Verification items for the finished model (mm, model axes). A direction names the side the tool comes from. Round coordinates to 2 decimals unless told otherwise and drop trailing zeros. Write each loop counter-clockwise with the first axis right and the second up, starting at its lowest first coordinate (ties: lowest second). Pieces come first, ordered by that corner, then holes. Notation, with made-up numbers: M 70,23 L 110,23 A8 cw 110,36 Z; hole C 54,68.25 d8. An arc over 180 degrees is marked long. One line per item, written item: value. Start each with the question number.
Item 1: Section check D-D, the plane z = -13.5. Record the cut outline in (x, y), then the cut area to 3 significant figures.
Item 2: Section check A-A, the plane y = 5.5. Record the cut outline in (x, z).
Item 3: Draft check along Z on faces 5 (the face through (10.99, 28.29, 20.64)), 6 (the face through (14, -14, 21)), 7 (the face through (5, -31, -17.35)). Enter one of: +Z half, -Z half, draft (parallel to the pull), parting line (faces both ways), or undercut.
Item 4: Gauge pin test, flat ends, axial feed: pin 1 (1 mm diameter, centred on y = 4, z = -8.5, fed in from +X); pin 2 (5 mm diameter, centred on x = 9.5, z = -18.5, fed in from -Y); pin 3 (1.4 mm diameter, centred on x = 7, z = 21.5, fed in from +Y); pin 4 (6 mm diameter, centred on y = -30.5, z = -21, fed in from -X). Record the tip position at first contact, or that the pin passes through.
Item 5: Tool access check on faces 1 (the face through (10.4, -30.4, 10.9)), 2 (the face through (10, 29.2, 21.4)), 3 (the face through (7, 31, -7)), 4 (the face through (7, 10, -3.9)). Record the directions out of +Z, -Z, +X, -X, +Y, -Y that give a thin tool (end or side, any length) a straight path to the whole face; none if there is none.
Item 6: Section check C-C, the plane y = 13.59. Record the cut outline in (x, z).
Item 7: Section check B-B, the plane z = 10.9. Record the cut outline in (x, y).
Item 8: Thickness scan on probe 1 along Y at (x, z) = (7.75, -8.5); probe 2 along Z at (x, y) = (4.5, 2); probe 3 along Z at (x, y) = (3.75, 12). Record the ranges inside material, lowest first. Write a range as from..to.
from build123d import *

# Parameters (mm, degrees)
SKETCH_1_W           = 46
SKETCH_1_H           = 64
EXTRUDE_1_DEPTH      = 12
SHELL_1_T            = -2
SKETCH_3_W           = 4.4
SKETCH_3_H           = 2
SKETCH_3_W_2         = 3.9
SKETCH_3_H_2         = 18.35
EXTRUDE_6_DEPTH      = 10
SKETCH_4_R           = 1
CUT_EXTRUDE_1_DEPTH  = 10
CUT_EXTRUDE_3_REACH  = 43.195
SKETCH_7_R           = 1
EXTRUDE_START        = -12
SKETCH_8_R           = 0.9
EXTRUDE_7_DEPTH      = 2
SKETCH_13_W          = 24
SKETCH_13_H          = 1.25
EXTRUDE_8_DEPTH      = 12
CUT_EXTRUDE_4_REACH  = 71.433
CUT_EXTRUDE_5_REACH  = 71.433
CUT_EXTRUDE_START    = -4
CUT_EXTRUDE_6_DEPTH  = 2.1
CUT_EXTRUDE_START_2  = -1.5
CUT_EXTRUDE_7_DEPTH  = 30.1
CUT_EXTRUDE_8_REACH  = 59.758
CUT_EXTRUDE_9_REACH  = 71.433
SKETCH_15_W          = 10
SKETCH_15_H          = 6
CUT_EXTRUDE_10_REACH = 59.758
SKETCH_16_W          = 1.6
SKETCH_16_H          = 6.7


with BuildPart() as part:
    # 草图1 → 凸台-拉伸1 (new body)
    with BuildSketch(Plane(origin=(0, 0, 0), x_dir=(0, 0, -1), z_dir=(1, 0, 0))):
        Rectangle(SKETCH_1_W, SKETCH_1_H)
    extrude(amount=EXTRUDE_1_DEPTH)

    # 抽壳1
    shell_1_openings = [part.faces().sort_by_distance(p)[0] for p in [
        (12, 0, 0),
    ]]
    offset(amount=SHELL_1_T, openings=shell_1_openings, kind=Kind.INTERSECTION)

    # 草图3 → 凸台-拉伸6 (add)
    # profile 1 of 5: a face of its own
    with BuildSketch(Plane(origin=(2, 0, 0), x_dir=(0, 0, -1), z_dir=(1, 0, 0))):
        with BuildLine():
            Line((20.175, -24.35), (21, -24.35))
            Line((21, -24.35), (21, -30))
            Line((21, -30), (15.35, -30))
            Line((15.35, -30), (15.35, -29.175))
            ThreePointArc((15.35, -29.175), (16.763209781, -25.763209781), (20.175, -24.35))
        make_face()
    # profile 2 of 5: a face of its own
    with BuildSketch(Plane(origin=(2, 0, 0), x_dir=(0, 0, -1), z_dir=(1, 0, 0))):
        with Locations((18.8, 1.6)):
            Rectangle(SKETCH_3_W, SKETCH_3_H)
    # profile 3 of 5: a face of its own
    with BuildSketch(Plane(origin=(2, 0, 0), x_dir=(0, 0, -1), z_dir=(1, 0, 0))):
        with BuildLine():
            Line((-21, 30), (-21, 24.35))
            Line((-21, 24.35), (-20.175, 24.35))
            ThreePointArc((-20.175, 24.35), (-17.207572663, 25.370397524), (-15.495256417, 28))
            Line((-15.495256417, 28), (-2, 28))
            Line((-2, 28), (-2, -2.35))
            Line((-2, -2.35), (5.9, -2.35))
            Line((5.9, -2.35), (5.9, 0.6))
            Line((5.9, 0.6), (10.4, 0.6))
            Line((10.4, 0.6), (10.4, 2.6))
            Line((10.4, 2.6), (5.9, 2.6))
            Line((5.9, 2.6), (5.9, 21.5))
            Line((5.9, 21.5), (0, 21.5))
            Line((0, 21.5), (0, 30))
            Line((0, 30), (-21, 30))
        make_face()
        with Locations((1.95, 10.325)):
            Rectangle(SKETCH_3_W_2, SKETCH_3_H_2, mode=Mode.SUBTRACT)
    # profile 4 of 5: a face of its own
    with BuildSketch(Plane(origin=(2, 0, 0), x_dir=(0, 0, -1), z_dir=(1, 0, 0))):
        with BuildLine():
            Line((-21, -10.7), (-21, -16.7))
            ThreePointArc((-21, -16.7), (-18, -13.7), (-21, -10.7))
        make_face()
    # profile 5 of 5: a face of its own
    with BuildSketch(Plane(origin=(2, 0, 0), x_dir=(0, 0, -1), z_dir=(1, 0, 0))):
        with BuildLine():
            Line((18.75, 30), (21, 30))
            Line((21, 30), (21, 27.9))
            Line((21, 27.9), (20.192225279, 27.9))
            ThreePointArc((20.192225279, 27.9), (19.145277228, 28.72622473), (18.75, 30))
        make_face()
    extrude(amount=EXTRUDE_6_DEPTH)

    # 草图4 → 切除-拉伸1 (cut)
    # profile 1 of 2: a face of its own
    with BuildSketch(Plane.ZY):
        with BuildLine():
            Line((-20.175, -26.35), (-23, -26.35))
            Line((-23, -26.35), (-23, -32))
            Line((-23, -32), (-17.382192318, -32))
            Line((-17.382192318, -32), (-17.35, -32))
            Line((-17.35, -32), (-17.35, -29.175))
            ThreePointArc((-17.35, -29.175), (-18.177423343, -27.177423343), (-20.175, -26.35))
        make_face()
        with Locations((-20.175, -29.175)):
            Circle(SKETCH_4_R, mode=Mode.SUBTRACT)
    # profile 2 of 2: a face of its own
    with BuildSketch(Plane.ZY):
        with BuildLine():
            Line((20.175, 26.35), (23, 26.35))
            Line((23, 26.35), (23, 32))
            Line((23, 32), (17.35, 32))
            Line((17.35, 32), (17.35, 29.175))
            ThreePointArc((17.35, 29.175), (18.177423343, 27.177423343), (20.175, 26.35))
        make_face()
        with Locations((20.175, 29.175)):
            Circle(SKETCH_4_R, mode=Mode.SUBTRACT)
    extrude(amount=-CUT_EXTRUDE_1_DEPTH, mode=Mode.SUBTRACT)

    # 草图7 → 切除-拉伸3 (cut, up to next)
    with BuildSketch(Plane.ZY, mode=Mode.PRIVATE) as cut_extrude_3_sk1:
        with Locations((-20.175, -29.175)):
            Circle(SKETCH_7_R)
    cut_extrude_3_tool1 = extrude(cut_extrude_3_sk1.sketch, amount=-CUT_EXTRUDE_3_REACH, mode=Mode.PRIVATE) & part.part
    # 草图7 → 切除-拉伸3 (cut, up to next)
    with BuildSketch(Plane.ZY, mode=Mode.PRIVATE) as cut_extrude_3_sk2:
        with Locations((20.175, 29.175)):
            Circle(SKETCH_7_R)
    cut_extrude_3_tool2 = extrude(cut_extrude_3_sk2.sketch, amount=-CUT_EXTRUDE_3_REACH, mode=Mode.PRIVATE) & part.part
    add(cut_extrude_3_tool1.solids().sort_by_distance((0, -29.175, -20.175))[0], mode=Mode.SUBTRACT)
    add(cut_extrude_3_tool2.solids().sort_by_distance((0, 29.175, 20.175))[0], mode=Mode.SUBTRACT)

    # 草图8 → 凸台-拉伸7 (add)
    with BuildSketch(Plane.ZY.offset(EXTRUDE_START)):
        with Locations(Location((-21, 30, 0), (0, 0, 180))):
            Circle(SKETCH_8_R)
        with Locations(Location((21, -13.7, 0), (0, 0, 180))):
            Circle(SKETCH_8_R)
    extrude(amount=-EXTRUDE_7_DEPTH)

    # 草图13 → 凸台-拉伸8 (add)
    with BuildSketch(Plane.ZY):
        with Locations((5, -29.375)):
            Rectangle(SKETCH_13_W, SKETCH_13_H)
    extrude(amount=-EXTRUDE_8_DEPTH)

    # 草图9 → 切除-拉伸4 (cut, up to next)
    with BuildSketch(Plane.XZ.offset(32), mode=Mode.PRIVATE) as cut_extrude_4_sk1:
        with BuildLine():
            Line((12, 9.3), (12, 12.5))
            ThreePointArc((12, 12.5), (10.4, 10.9), (12, 9.3))
        make_face()
    cut_extrude_4_tool1 = extrude(cut_extrude_4_sk1.sketch, amount=-CUT_EXTRUDE_4_REACH, mode=Mode.PRIVATE) & part.part
    add(cut_extrude_4_tool1.solids().sort_by_distance((11.320939, -32, 10.9))[0], mode=Mode.SUBTRACT)

    # 草图11 → 切除-拉伸5 (cut, up to next)
    with BuildSketch(Plane(origin=(0, 32, 0), x_dir=(1, 0, 0), z_dir=(0, 1, 0)), mode=Mode.PRIVATE) as cut_extrude_5_sk1:
        with BuildLine():
            Line((12, 12.4), (12, 14.6))
            ThreePointArc((12, 14.6), (10.9, 13.5), (12, 12.4))
        make_face()
    cut_extrude_5_tool1 = extrude(cut_extrude_5_sk1.sketch, amount=-CUT_EXTRUDE_5_REACH, mode=Mode.PRIVATE) & part.part
    add(cut_extrude_5_tool1.solids().sort_by_distance((11.533146, 32, -13.5))[0], mode=Mode.SUBTRACT)

    # 草图12 → 切除-拉伸6 (cut)
    with BuildSketch(Plane(origin=(0, 32, 0), x_dir=(1, 0, 0), z_dir=(0, 1, 0)).offset(CUT_EXTRUDE_START)):
        with BuildLine():
            Line((12, -12.5), (12, -9.3))
            ThreePointArc((12, -9.3), (10.4, -10.9), (12, -12.5))
        make_face()
    extrude(amount=CUT_EXTRUDE_6_DEPTH, mode=Mode.SUBTRACT)

    # 草图10 → 切除-拉伸7 (cut)
    with BuildSketch(Plane.XZ.offset(32).offset(CUT_EXTRUDE_START_2)):
        with BuildLine():
            Line((12, -2.4), (12, -0.2))
            ThreePointArc((12, -0.2), (10.9, -1.3), (12, -2.4))
        make_face()
    extrude(amount=-CUT_EXTRUDE_7_DEPTH, mode=Mode.SUBTRACT)

    # 草图14 → 切除-拉伸8 (cut, up to next)
    with BuildSketch(Plane.XY.offset(23), mode=Mode.PRIVATE) as cut_extrude_8_sk1:
        with BuildLine():
            Line((12, 17.79), (12, 9.39))
            ThreePointArc((12, 9.39), (7.8, 13.59), (12, 17.79))
        make_face()
    cut_extrude_8_tool1 = extrude(cut_extrude_8_sk1.sketch, amount=-CUT_EXTRUDE_8_REACH, mode=Mode.PRIVATE) & part.part
    add(cut_extrude_8_tool1.solids().sort_by_distance((10.217465, 13.59, 23))[0], mode=Mode.SUBTRACT)

    # 草图15 → 电机线切除-拉伸9 (cut, up to next)
    with BuildSketch(Plane(origin=(0, 32, 0), x_dir=(1, 0, 0), z_dir=(0, 1, 0)), mode=Mode.PRIVATE) as cut_extrude_9_sk1:
        with Locations((7, 4)):
            Rectangle(SKETCH_15_W, SKETCH_15_H)
    cut_extrude_9_tool1 = extrude(cut_extrude_9_sk1.sketch, amount=-CUT_EXTRUDE_9_REACH, mode=Mode.PRIVATE) & part.part
    add(cut_extrude_9_tool1.solids().sort_by_distance((7, 32, -4))[0], mode=Mode.SUBTRACT)

    # 草图16 → 拨杆切除-拉伸10 (cut, up to next)
    with BuildSketch(Plane.XY.offset(23), mode=Mode.PRIVATE) as cut_extrude_10_sk1:
        with Locations((11.2, -21.55)):
            Rectangle(SKETCH_16_W, SKETCH_16_H)
    cut_extrude_10_tool1 = extrude(cut_extrude_10_sk1.sketch, amount=-CUT_EXTRUDE_10_REACH, mode=Mode.PRIVATE) & part.part
    add(cut_extrude_10_tool1.solids().sort_by_distance((11.2, -21.55, 23))[0], mode=Mode.SUBTRACT)


solid = part.part
Response values:
1. outline: M 0,-32 L 12,-32 L 12,-30 L 2,-30 L 2,30 L 10.9,30 L 10.9,32 L 0,32 Z
1. area: 166 mm2
2. outline: M 0,-23 L 12,-23 L 12,-21 L 2,-21 L 2,-5.9 L 12,-5.9 L 12,-3.9 L 2,-3.9 L 2,0 L 12,0 L 12,2 L 2,2 L 2,21 L 12,21 L 12,23 L 0,23 Z
3. face 5: undercut
3. face 6: draft
3. face 7: -Z half
4. pin 1: stops at x = 2
4. pin 2: stops at y = -32
4. pin 3: stops at y = 26.35
4. pin 4: stops at x = 10
5. face 1: +X, -Y
5. face 2: +Z, -X, +Y
5. face 3: +X, +Y
5. face 4: +X
6. outline: M 0,-23 L 12,-23 L 12,-21 L 2,-21 L 2,-5.9 L 12,-5.9 L 12,-3.9 L 2,-3.9 L 2,0 L 12,0 L 12,2 L 2,2 L 2,21 L 7.8,21 L 7.8,23 L 0,23 Z
7. outline: M 0,-32 L 10.4,-32 L 10.4,-28.75 L 2,-28.75 L 2,28 L 10.4,28 L 10.4,30.1 L 12,30.1 L 12,32 L 0,32 Z
8. probe 1: y = -32..-30, 0.6..2.6, 30..32
8. probe 2: z = -23..-16.6, -10.4..-3.9, 0..2, 21..23
8. probe 3: z = -23..-21, -5.9..-3.9, 0..2, 21..23
